Input: part model. Units: mm. Frame: model coordinates. A direction names the side the tool comes from. Give positions to 0.01 mm unless a question says otherwise; leave off trailing zeros. Loops run counter-clockwise (first coordinate to the right, second up) from the corner with the lowest first, then second, coordinate; pieces in that order, holes last. Notation, with made-up numbers: (86.25, -19.5) - (143.25, -19.5) arc R18 cw to (143.25, 10.5) - close; hole circle Ø5 at (36.25, 1). An arc over 180 degrees is marked (long way). Answer as a JSON object with one key per item and string values.
from build123d import *

# Parameters (mm, degrees)
CUT_EXTRUDE_1_REACH = 22
SKETCH_2_R          = 3


with BuildPart() as part:
    # 草图1 → 旋转1 (revolve)
    with BuildSketch(Plane(origin=(0, 0, 0), x_dir=(1, 0, 0), z_dir=(0, 1, 0))):
        Polygon((0, 30), (0, 43.5), (8, 43.5), (8, 27), (20, 27), (20, 19), (17, 19), (17, 21), (3, 21), (3, 30), align=None)
    revolve(axis=Axis((0, 0, 0), (1, 0, 0)))

    # 草图2 → 切除-拉伸1 (cut, up to next)
    with BuildSketch(Plane.ZY, mode=Mode.PRIVATE) as cut_extrude_1_sk1:
        with Locations((0, -37.5)):
            Circle(SKETCH_2_R)
    cut_extrude_1_tool1 = extrude(cut_extrude_1_sk1.sketch, amount=-CUT_EXTRUDE_1_REACH, mode=Mode.PRIVATE) & part.part
    add(cut_extrude_1_tool1.solids().sort_by_distance((0, -37.5, 0))[0], mode=Mode.SUBTRACT)
    # 草图2 → 切除-拉伸1 (cut, up to next)
    with BuildSketch(Plane.ZY, mode=Mode.PRIVATE) as cut_extrude_1_sk2:
        with Locations((0, 37.5)):
            Circle(SKETCH_2_R)
    cut_extrude_1_tool2 = extrude(cut_extrude_1_sk2.sketch, amount=-CUT_EXTRUDE_1_REACH, mode=Mode.PRIVATE) & part.part
    add(cut_extrude_1_tool2.solids().sort_by_distance((0, 37.5, 0))[0], mode=Mode.SUBTRACT)
    # 草图2 → 切除-拉伸1 (cut, up to next)
    with BuildSketch(Plane.ZY, mode=Mode.PRIVATE) as cut_extrude_1_sk3:
        with Locations((-37.5, 0)):
            Circle(SKETCH_2_R)
    cut_extrude_1_tool3 = extrude(cut_extrude_1_sk3.sketch, amount=-CUT_EXTRUDE_1_REACH, mode=Mode.PRIVATE) & part.part
    add(cut_extrude_1_tool3.solids().sort_by_distance((0, 0, -37.5))[0], mode=Mode.SUBTRACT)
    # 草图2 → 切除-拉伸1 (cut, up to next)
    with BuildSketch(Plane.ZY, mode=Mode.PRIVATE) as cut_extrude_1_sk4:
        with Locations((37.5, 0)):
            Circle(SKETCH_2_R)
    cut_extrude_1_tool4 = extrude(cut_extrude_1_sk4.sketch, amount=-CUT_EXTRUDE_1_REACH, mode=Mode.PRIVATE) & part.part
    add(cut_extrude_1_tool4.solids().sort_by_distance((0, 0, 37.5))[0], mode=Mode.SUBTRACT)


solid = part.part
Item 1: Cut plane C-C (z = 37.5). Return loops of the section in (x, y), then the cut area to 3 significant figures.
Geometry check:
{"outline": "(0, -22.05) - (8, -22.05) - (8, -3) - (0, -3) - close; (0, 3) - (8, 3) - (8, 22.05) - (0, 22.05) - close", "area": "305 mm2"}
Item 2: Access query for faces 1 (the face through (3.944, -34.526, -0.391)), 2 (the face through (3, 20.4, 6.2)), 3 (the face through (8, -19, 20)). Directions: +Z, -Z, +X, -X, +Y, -Y. A direction counts if a zero-diameter tool reaches every point of the face in a straight line with its end or side. Return the directions, or none.
Geometry check:
{"face 1": "+X, -X", "face 2": "-X", "face 3": "+X"}
Item 3: Material intervals for line 1 (Y direction, x = 4, z = 0); line 2 (Y direction, x = 2, z = 0); line 3 (Y direction, x = 19.1, z = 0), sorted ascending. Write a range as [from, to].
Geometry check:
{"line 1": "y = [-43.5, -40.5], [-34.5, -21], [21, 34.5], [40.5, 43.5]", "line 2": "y = [-43.5, -40.5], [-34.5, -30], [30, 34.5], [40.5, 43.5]", "line 3": "y = [-27, -19], [19, 27]"}
Item 4: Mould query, pull axis Z, two halves, no side actions, for faces 4 (the face through (9.9, 6.31, -20.03)), 5 (the face through (14.08, -26.36, 5.85)), 6 (the face through (0, -28.4, -10.3)). Classes: released by +Z, released by -Z, zero draft, split by the parting line, or undercut.
Geometry check:
{"face 4": "undercut", "face 5": "split by the parting line", "face 6": "zero draft"}
Item 5: Contact query for flat-ended pins moving along their axis: P1, Ø8, axis at x = 7, y = 24.5, coming from the +Z side; P2, Ø1, axis at x = 13.5, z = 0.5, coming from the -Y side; P3, Ø1.5, axis at y = -10.5, z = -33.5, coming from the +X side. Output: stop coordinate, or through.
Geometry check:
{"P1": "stops at z = 38.37", "P2": "stops at y = -27", "P3": "stops at x = 8"}
Item 6: Cut plane D-D (x = 6.75). Return loops of the section in (y, z).
Geometry check:
{"outline": "circle Ø87 at (0, 0); hole circle Ø6 at (-37.5, 0); hole circle Ø42 at (0, 0); hole circle Ø6 at (0, -37.5); hole circle Ø6 at (0, 37.5); hole circle Ø6 at (37.5, 0)"}
Item 7: Cut plane A-A (y = 0). Return loops of the section in (x, z), then the cut area to 3 significant figures.
Geometry check:
{"outline": "(0, -43.5) - (8, -43.5) - (8, -40.5) - (0, -40.5) - close; (0, -34.5) - (8, -34.5) - (8, -27) - (20, -27) - (20, -19) - (17, -19) - (17, -21) - (3, -21) - (3, -30) - (0, -30) - close; (0, 30) - (3, 30) - (3, 21) - (17, 21) - (17, 19) - (20, 19) - (20, 27) - (8, 27) - (8, 34.5) - (0, 34.5) - close; (0, 40.5) - (8, 40.5) - (8, 43.5) - (0, 43.5) - close", "area": "366 mm2"}
